from build123d import *

# Parameters (mm, degrees)
SKETCH2_R           = 5
SKETCH2_R_2         = 10
BOSS_EXTRUDE2_DEPTH = 10
SKETCH3_R           = 15
SKETCH3_R_2         = 10
BOSS_EXTRUDE3_DEPTH = 20
SKETCH4_R           = 2.5
SKETCH4_R_2         = 15
BOSS_EXTRUDE5_DEPTH = 5
SKETCH5_R           = 15
SKETCH5_R_2         = 10
BOSS_EXTRUDE6_DEPTH = 50


with BuildPart() as part:
    # Sketch2 → Boss-Extrude2 (new body)
    with BuildSketch(Plane(origin=(0, 0, 0), x_dir=(0, 0, -1), z_dir=(1, 0, 0))):
        with BuildLine():
            ThreePointArc((9.684825363, 44.990814664), (8e-08, 52.5), (-9.684825323, 44.990814819))
            add(Edge.make_bspline(
                [(-40.752503599, -12.061652047), (-20.934905138, 4.420586079), (-10.579005904, 23.438067717), (-9.684825323, 44.990814819)],
                knots=[0, 0, 0, 0, 0.868352025, 0.868352025, 0.868352025, 0.868352025], degree=3))
            ThreePointArc((-40.752503599, -12.061652047), (-45.466333468, -26.2500004), (-30.821948144, -29.261876808))
            add(Edge.make_bspline(
                [(-30.821948144, -29.261876808), (1.426149217, -20.445917502), (30.821948237, -29.261876878)],
                knots=[0, 0, 0, 0.907199698, 0.907199698, 0.907199698], degree=2))
            ThreePointArc((30.821948237, -29.261876878), (45.466333568, -26.250000227), (40.752503338, -12.061651935))
            add(Edge.make_bspline(
                [(40.752503338, -12.061651935), (11.072313354, 12.162082971), (9.684825363, 44.990814664)],
                knots=[0, 0, 0, 1, 1, 1], degree=2))
        make_face()
        with Locations((0, 42.5)):
            Circle(SKETCH2_R, mode=Mode.SUBTRACT)
        with Locations((36.806079661, -21.25)):
            Circle(SKETCH2_R, mode=Mode.SUBTRACT)
        with Locations((-36.806079661, -21.25)):
            Circle(SKETCH2_R, mode=Mode.SUBTRACT)
        Circle(SKETCH2_R_2, mode=Mode.SUBTRACT)
    extrude(amount=BOSS_EXTRUDE2_DEPTH)

    # Sketch3 → Boss-Extrude3 (add)
    with BuildSketch(Plane(origin=(10, 0, 0), x_dir=(0, 0, -1), z_dir=(1, 0, 0))):
        Circle(SKETCH3_R)
        Circle(SKETCH3_R_2, mode=Mode.SUBTRACT)
    extrude(amount=BOSS_EXTRUDE3_DEPTH)

    # Sketch4 → Boss-Extrude5 (add)
    with BuildSketch(Plane(origin=(30, 0, 0), x_dir=(0, 0, -1), z_dir=(1, 0, 0))):
        with BuildLine():
            ThreePointArc((21.488966336, 6.668907393), (23.815698604, 13.75), (16.519926386, 15.275537051))
            ThreePointArc((16.519926386, 15.275537051), (0, 22.5), (-16.519926386, 15.275537051))
            ThreePointArc((-16.519926386, 15.275537051), (-23.815698604, 13.75), (-21.488966336, 6.668907393))
            ThreePointArc((-21.488966336, 6.668907393), (-22.5, 0), (-21.488966336, -6.668907393))
            ThreePointArc((-21.488966336, -6.668907393), (-23.815698604, -13.75), (-16.519926386, -15.275537051))
            ThreePointArc((-16.519926386, -15.275537051), (0, -22.5), (16.519926386, -15.275537051))
            ThreePointArc((16.519926386, -15.275537051), (23.815698604, -13.75), (21.488966336, -6.668907393))
            ThreePointArc((21.488966336, -6.668907393), (22.5, 0), (21.488966336, 6.668907393))
        make_face()
        with Locations((19.485571585, 11.25)):
            Circle(SKETCH4_R, mode=Mode.SUBTRACT)
        with Locations((19.485571585, -11.25)):
            Circle(SKETCH4_R, mode=Mode.SUBTRACT)
        with Locations((-19.485571585, -11.25)):
            Circle(SKETCH4_R, mode=Mode.SUBTRACT)
        with Locations((-19.485571585, 11.25)):
            Circle(SKETCH4_R, mode=Mode.SUBTRACT)
        Circle(SKETCH4_R_2, mode=Mode.SUBTRACT)
    extrude(amount=-BOSS_EXTRUDE5_DEPTH)

    # Sketch5 → Boss-Extrude6 (add)
    with BuildSketch(Plane(origin=(30, 0, 0), x_dir=(0, 0, -1), z_dir=(1, 0, 0))):
        Circle(SKETCH5_R)
        Circle(SKETCH5_R_2, mode=Mode.SUBTRACT)
    extrude(amount=BOSS_EXTRUDE6_DEPTH)


solid = part.part
Can you work these out from the model? Positions are in its coordinate system, mm. A direction names the side the tool comes from. Coordinates: 2 decimals unless noted, no trailing zeros. Order: outer loops, then holes, each group sorted by start corner. A loop starts at its lowest first (then second) coordinate and runs counter-clockwise, first axis right, second up. Notation, with made-up numbers: M 70.5,80 L 81.5,80 A11 ccw 81.5,101 Z; hole C -1.5,-25 d4. An arc over 180 degrees is marked long. Write item = value, one per line.
(1) If we mould it in two halves opening along Y, with no side actions, what happens to faces 1 (the face through (27.5, 22.5, -0.3)), 2 (the face through (17.395, 0.66, 14.985)), 3 (the face through (27.5, 13.6, -23.9)), 4 (the face through (39.44, -9.76, 2.17))? For each: pulls with the +Y half, pulls with the -Y half, needs draft (parallel to the pull), parting line crosses it, or undercut.
Results are:
face_1 = pulls with the +Y half
face_2 = parting line crosses it
face_3 = undercut
face_4 = undercut
(2) I need wall thicknesses on line 1 along Y through (x, z) = (3, 0); line 2 along Z through (x, y) = (28, 11); line 3 along X through (y, z) = (5.5, 18). Which ranges of each line are inside material? Lowest first, please. Write a range as [from, to].
Results are:
line_1 = [-24.86, -10], [10, 37.5], [47.5, 52.5]
line_2 = [-24.48, -21.97], [-17, 17], [21.97, 24.48]
line_3 = [0, 10], [25, 30]
(3) For pin 1 Ø5 at (x, y) = (42.5, 6.5) entering from +Z; pin 2 Ø13 at (y, z) = (42.5, 0) entering from -X; pin 3 Ø18 at (y, z) = (0, 0) entering from -X; pin 4 Ø5 at (x, y) = (22, -16) entering from -Z, each with a flat end and sliding along its axis, tell me the tip position at first contact or that it passes through.
Results are:
pin_1 = 14.46
pin_2 = 0
pin_3 = through
pin_4 = -6.54
(4) Suppose I cut it at C-C on x = 11.5. Please give me the cut outline in (y, z), plus the area to 3 significant figures.
Results are:
outline = C 0,0 d30; hole C 0,0 d20
area = 393 mm2
(5) Suppose I cut it at D-D on z = 0. State how many separate pieces and enclosed holes the cut face has, plus the area to 3 significant figures.
Results are:
separate_pieces = 3
enclosed_holes = 0
area = 1,250 mm2
(6) Suppose I cut it at A-A on x = 27. Please give me the cut outline in (y, z).
Results are:
outline = M -15.28,-16.52 A5 ccw long -6.67,-21.49 A22.5 ccw 6.67,-21.49 A5 ccw long 15.28,-16.52 A22.5 ccw 15.28,16.52 A5 ccw long 6.67,21.49 A22.5 ccw -6.67,21.49 A5 ccw long -15.28,16.52 A22.5 ccw Z; hole C -11.25,-19.49 d5; hole C -11.25,19.49 d5; hole C 0,0 d20; hole C 11.25,-19.49 d5; hole C 11.25,19.49 d5
(7) For faces 5 (the face through (27.5, -13.6, 23.9)), 6 (the face through (25, 10.3, 11.2)), 7 (the face through (27.5, -22.5, 0.3)), which set-ups out of +Z, -Z, +X, -X, +Y, -Y let a thin tool reach every point of the face, with its end or its side?
Results are:
face_5 = +X
face_6 = none
face_7 = +X, -Y
(8) Suppose I cut it at B-B on y = -21.25. Please give me the cut outline in (x, z).
Results are:
outline = M 0,-46.81 L 10,-46.81 L 10,-41.81 L 0,-41.81 Z; M 0,-31.81 L 10,-31.81 L 10,31.81 L 0,31.81 Z; M 0,41.81 L 10,41.81 L 10,46.81 L 0,46.81 Z; M 25,-7.4 L 30,-7.4 L 30,7.4 L 25,7.4 Z
